Source: three-view drawing plus pictorial views. Frame: mm from the lowest corner of the part. Give positions to 0.01 mm unless a question says otherwise; leave off trailing zeros. Loops run counter-clockwise (first coordinate to the right, second up) from the corner with the lowest first, then second, coordinate; pieces in that order, holes last. Notation, with made-up numbers: (29, 0.5) - (44, 0.5) arc R10 ccw to (44, 9.5) - close; hole circle Ø2 at (-23.75, 45.25). An arc over 180 degrees is marked (long way). Answer in a Markdown table with one row per item.
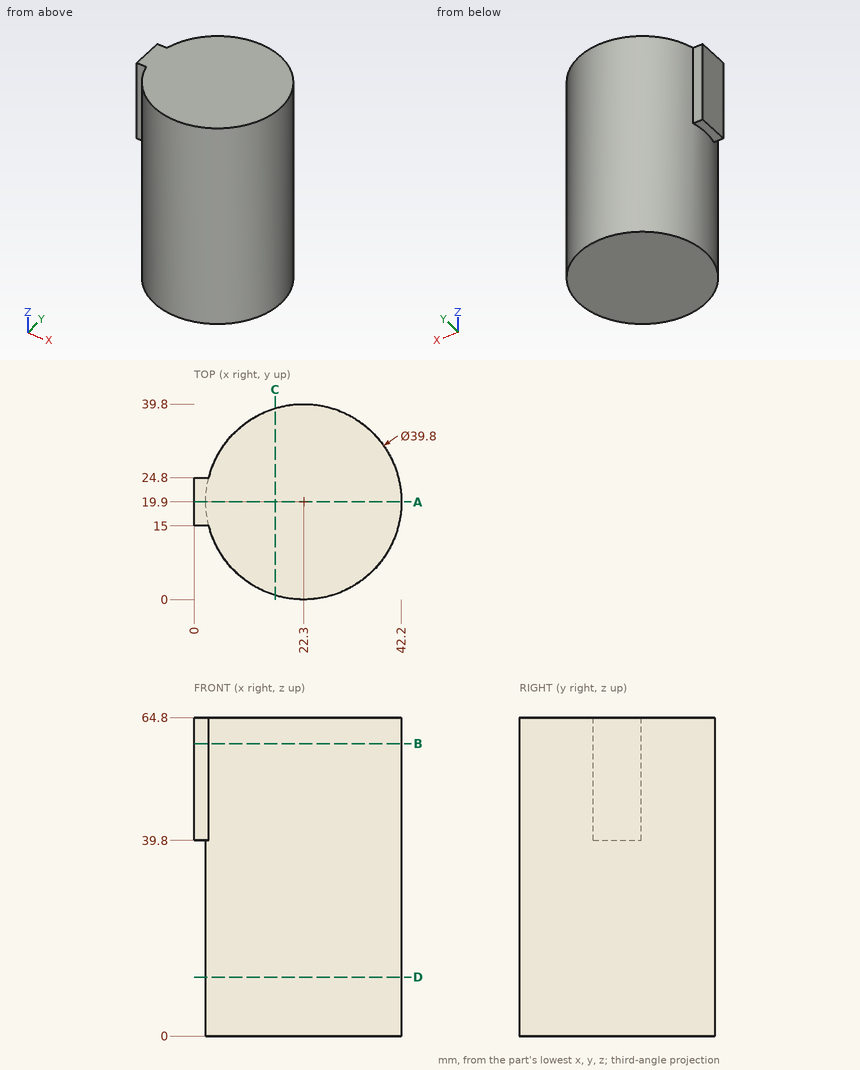
Q1. Cut plane D-D (z = 12). Output: boundary loops of the cut face in (x, y), and give its area (3 significant figures).
Check values:
| item | result |
|---|---|
| outline | circle Ø39.8 at (22.3, 19.9) |
| area | 1,240 mm² |
Q2. Material intervals for line 1 along Y through (x, z) = (11, 41); line 2 along X through (y, z) = (19, 24.5); line 3 along Y through (x, z) = (4, 8), sorted ascending.
Check values:
| item | result |
|---|---|
| line 1 | 3.52 to 36.28 |
| line 2 | 2.42 to 42.18 |
| line 3 | 12.08 to 27.72 |
Q3. Cut plane C-C (x = 16.5). Output: boundary loops of the cut face in (y, z).
Check values:
| item | result |
|---|---|
| outline | (0.86, 0) - (38.94, 0) - (38.94, 64.8) - (0.86, 64.8) - close |
Q4. Cut plane B-B (z = 59.5). Output: boundary loops of the cut face in (x, y), and give its area (3 significant figures).
Check values:
| item | result |
|---|---|
| outline | (0, 15) - (3.01, 15) arc R19.9 ccw (long way) to (3.01, 24.8) - (0, 24.8) - close |
| area | 1,270 mm² |
Q5. First-contact query: pin 1 (5 mm diameter, centred on y = 29.5, z = 27.5, fed in from +X); pin 2 (3 mm diameter, centred on y = 30, z = 20.5, fed in from +X); pin 3 (1 mm diameter, centred on x = 19.5, z = 43.5, fed in from +Y). Flat tips, straight axial feed; report the tip coordinate or a pass-through.
Check values:
| item | result |
|---|---|
| pin 1 | x = 40.89 |
| pin 2 | x = 40.25 |
| pin 3 | y = 39.67 |
Q6. Cut plane A-A (y = 19.9). Output: boundary loops of the cut face in (x, z), and give its area (3 significant figures).
Check values:
| item | result |
|---|---|
| outline | (0, 39.8) - (2.4, 39.8) - (2.4, 0) - (42.2, 0) - (42.2, 64.8) - (0, 64.8) - close |
| area | 2,640 mm² |
